```python
from build123d import *

# Parameters (mm, degrees)
SKETCH_1_W      = 248.5
SKETCH_1_H      = 200
SKETCH_1_R      = 2.5
EXTRUDE_1_DEPTH = 0.5


with BuildPart() as part:
    # 스케치1 → 보스-돌출1 (new, symmetric)
    with BuildSketch(Plane.XY):
        with Locations((124.25, 100)):
            Rectangle(SKETCH_1_W, SKETCH_1_H)
        with Locations((124.25, 11)):
            Circle(SKETCH_1_R, mode=Mode.SUBTRACT)
        with Locations((204.25, 11)):
            Circle(SKETCH_1_R, mode=Mode.SUBTRACT)
        with Locations((44.25, 11)):
            Circle(SKETCH_1_R, mode=Mode.SUBTRACT)
    extrude(amount=EXTRUDE_1_DEPTH, both=True)


solid = part.part
```
The model under review builds one solid part; all positions refer to its coordinate system, in mm. Coordinates: 2 decimals unless noted, no trailing zeros. One line per item, written item: value. Start each with the question number.
Q1. To check wall thickness, follow probe 1 along Y at (x, z) = (44.25, -0.25); probe 2 along Y at (x, z) = (123.5, -0.3). State the ranges of each line that lie inside material, in increasing order.
Q2. Clearance check with a flat-ended pin moving along its axis: P1, Ø4, axis at x = 44.25, y = 11, coming from the -Z side. State where the tip first meets the part, or that it passes through.
Q3. The part is to be moulded in two halves that separate along X. For faces 1 (the face through (123, 101, 0.5)), 2 (the face through (126.635, 11.751, -0.007)), say which applies: +X half, -X half, draft (parallel to the pull), parting line (faces both ways), or undercut.
Response:
1. probe 1: 0 to 8.5, 13.5 to 200
1. probe 2: 0 to 8.62, 13.38 to 200
2. P1: through
3. face 1: draft
3. face 2: undercut
